Part print with two shaded views. Sizes in mm from the minimum x, y, z corner. A direction names the side the tool comes from. Give positions to 0.01 mm unless a question says otherwise; leave off trailing zeros. Write each loop counter-clockwise with the first axis right and the second up, starting at its lowest first coordinate (ties: lowest second). Pieces come first, ordered by that corner, then holes. Notation, with made-up numbers: M 32,71.5 L 80,71.5 A23 ccw 80,80.5 Z; hole C 49,3 d4. An arc over 180 degrees is marked long. One line per item, written item: value. Start each with the question number.
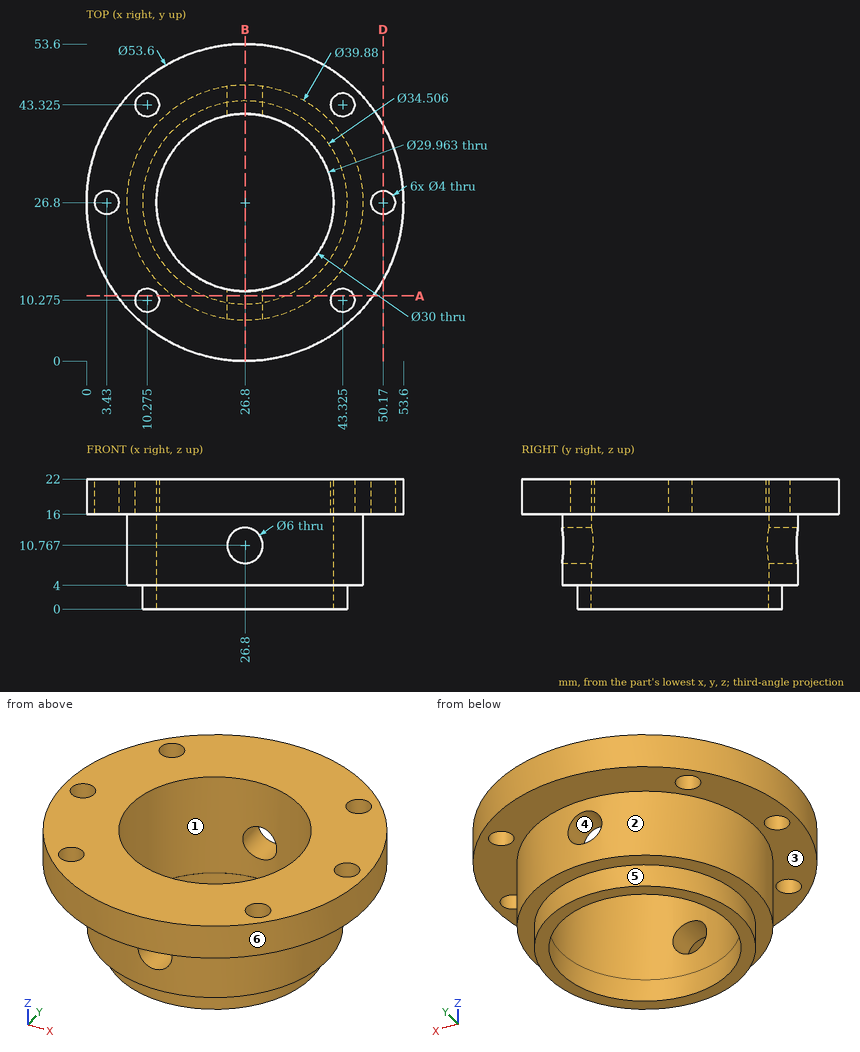
1) Tool access for the marked faces 5 and 6: list every direction of +Z, -Z, +X, -X, +Y, -Y with a clear straight run to the whole face (end or side of a thin tool).
2) Band-saw the part on A-A (y = 11). List the corners of the cut face in (x, z) (1 decimal).
3) Probe line 1 along Y through (x, z) = (26.8, 2.9); line 2 along Z through (x, y) = (15, 46.5); line 3 along Z through (x, y) = (7, 25.5). List the from-to ranges inside material, lowest first. Write a range as from..to.
4) Drop flat-ended pins along their axis: P1, Ø9.5, axis at x = 26.8, z = 10.77, coming from the +Y side; P2, Ø24, axis at x = 26.8, y = 26.8, coming from the -Z side (1 decimal); P3, Ø7, axis at x = 26.8, z = 10.77, coming from the -Y side; P4, Ø3, axis at x = 45, z = 5.5, coming from the -Y side (1 decimal). Give the stop position or say it passes through.
5) Band-saw the part on D-D (x = 50.17). List the corners of the cut face in (y, z).
6) Band-saw the part on B-B (x = 26.8). Count the separate pieces of the cut face and the enclosed holes in it, then the cut area to 3 significant figures.
7) Mould opens along X. For the marked faces 1, 2, 3 and 4 say: released by +X, released by -X, zero draft, split by the parting line, or undercut.
Model answer:
1. face 5: -Z
1. face 6: +Z, -Z
2. outline: M 5.2,16 L 8.4,16 L 8.4,22 L 5.2,22 Z; M 12.1,16 L 14.6,16 L 14.6,4 L 19.9,4 L 19.9,0 L 33.7,0 L 33.7,4 L 39,4 L 39,16 L 41.5,16 L 41.5,22 L 12.1,22 Z; M 45.2,16 L 48.4,16 L 48.4,22 L 45.2,22 Z; hole C 26.8,10.8 d6
3. line 1: y = 9.55..11.82, 41.78..44.05
3. line 2: z = 16..22
3. line 3: z = 4..22
4. P1: stops at y = 46.74
4. P2: passes through
4. P3: stops at y = 6.86
4. P4: stops at y = 15.9
5. outline: M 13.68,16 L 24.8,16 L 24.8,22 L 13.68,22 Z; M 28.8,16 L 39.92,16 L 39.92,22 L 28.8,22 Z
6. separate pieces: 4
6. enclosed holes: 0
6. area: 219 mm²
7. face 1: undercut
7. face 2: split by the parting line
7. face 3: zero draft
7. face 4: undercut
